Here's how the part is built. I have some questions about the finished solid (model axes, mm). Face numbers are marked on the shaded views. A direction names the side the tool comes from. Give positions to 0.01 mm unless a question says otherwise; leave off trailing zeros. Write each loop counter-clockwise with the first axis right and the second up, starting at its lowest first coordinate (ties: lowest second). Pieces come first, ordered by that corner, then holes. Notation, with made-up numbers: (2, 20) - (60, 20) arc R22 ccw to (60, 59) - close; hole circle Ø7 at (-9, -15.75). An arc over 180 degrees is marked (long way). Write each question's results on one line, items separated by ' | '. Start each with the question number.
Item 1: Suppose I cut it at C-C on z = -59. List the corners of the cut face in (x, y) for me.
Item 2: Which directions (+Z, -Z, +X, -X, +Y, -Y) give clear straight access to the entire face, cutting with the end or side of a thin tool? Please do the marked faces 4 and 5.
Item 3: We'd pull the mould along Y, two halves only. Please class the marked faces 1, 2 and 3: +Y half, -Y half, draft (parallel to the pull), parting line (faces both ways), or undercut.
Item 4: Suppose I cut it at B-B on y = 62. List the corners of the cut face in (x, z) for me.
Item 5: Please list where these lines run through material, in increasing order: line 1 along Y through (x, z) = (13.5, -72); line 2 along X through (y, z) = (57, -7); line 3 along Z through (x, y) = (74.5, 80).
Item 6: Suppose I cut it at A-A on x = 39.5. List the corners of the cut face in (y, z) for me, then the cut area to 3 significant figures.
```python
from build123d import *

# Parameters (mm, degrees)
BOSS_EXTRUDE1_DEPTH = 84
SKETCH2_W           = 78
SKETCH2_H           = 12.96225643
CUT_EXTRUDE1_DEPTH  = 157.847059265


with BuildPart() as part:
    # Sketch1 → Boss-Extrude1 (new body)
    with BuildSketch(Plane(origin=(0, 0, 0), x_dir=(0, 0, -1), z_dir=(1, 0, 0))):
        Polygon((0, 0), (0, 78), (13, 88), (99, 88), (99, 0), align=None)
    extrude(amount=BOSS_EXTRUDE1_DEPTH)

    # Sketch2 → Cut-Extrude1 (cut, through all)
    with BuildSketch(Plane(origin=(0, 0, -99), x_dir=(-1, 0, 0), z_dir=(0, 0, -1))):
        with Locations((-42, 58)):
            Rectangle(SKETCH2_W, SKETCH2_H)
    extrude(amount=-CUT_EXTRUDE1_DEPTH, mode=Mode.SUBTRACT)


solid = part.part
```
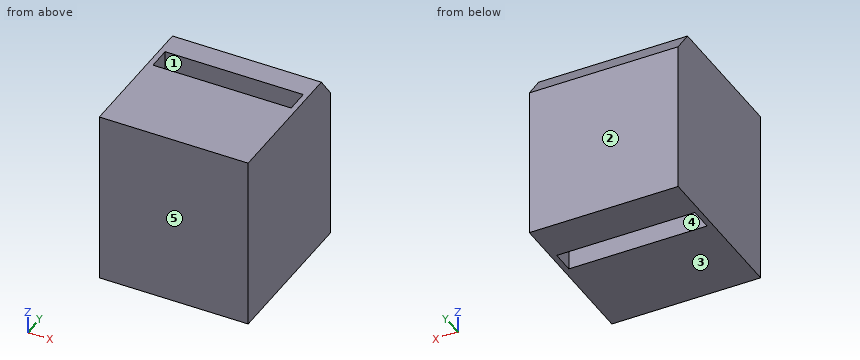
Checked values:
1) outline: (0, 0) - (84, 0) - (84, 88) - (0, 88) - close; hole (3, 51.52) - (81, 51.52) - (81, 64.48) - (3, 64.48) - close
2) face 4: +Z, -Z | face 5: +Z, -Z, +X, -X, -Y
3) face 1: undercut | face 2: +Y half | face 3: draft
4) outline: (0, -99) - (3, -99) - (3, 0) - (0, 0) - close; (81, -99) - (84, -99) - (84, 0) - (81, 0) - close
5) line 1: y = 0 to 51.52, 64.48 to 88 | line 2: x = 0 to 3, 81 to 84 | line 3: z = -99 to -2.6
6) outline: (0, -99) - (51.52, -99) - (51.52, 0) - (0, 0) - close; (64.48, -99) - (88, -99) - (88, -13) - (78, 0) - (64.48, 0) - close | area: 7,360 mm^2
